The model under review builds one solid part; all positions refer to its coordinate system, in mm. Face numbers are marked on the shaded views. Coordinates: 2 decimals unless noted, no trailing zeros. Write each loop counter-clockwise with the first axis right and the second up, starting at its lowest first coordinate (ties: lowest second). Pieces come first, ordered by that corner, then holes. Notation, with made-up numbers: (28.25, 24.25) - (73.25, 24.25) arc R20 ccw to (73.25, 57.25) - close; hole circle Ø9 at (-4.75, -16.5). An arc over 180 degrees is marked (long way). Put each result on its own line as item: value. Start each with the question number.
Item 1: Consider section D-D on y = 3.5. Give the boundary of the cut face in (x, z).
Item 2: Consider section A-A on y = 1.75. Give the boundary of the cut face in (x, z).
Item 3: To check wall thickness, follow L1, parallel to Y at x = 0, z = 0.5; L2, parallel to X at y = -1, z = 2; L3, parallel to X at y = -0.5, z = 1.5. State the ranges of each line that lie inside material, in increasing order. Write a range as [from, to].
Item 4: For pin 1 (1 mm diameter, centred on y = -2, z = 1, fed in from +X), flat-tipped, find the tip position at first contact; note if it passes through.
Item 5: Consider section B-B on y = 0. Give the boundary of the cut face in (x, z).
Item 6: Mouldability with a two-part tool opening along X and no side actions: class the marked faces 1, 2 and 3 as pulls with the +X half, pulls with the -X half, needs draft (parallel to the pull), parting line crosses it, or undercut.
Item 7: Consider section C-C on x = 17.5. Give the boundary of the cut face in (y, z), then the cut area to 3 significant figures.
```python
from build123d import *

# Parameters (mm, degrees)
BOSS_EXTRUDE1_DEPTH     = 3.556
CUT_EXTRUDE1_DEPTH      = 23.127926609
CUT_EXTRUDE1_DEPTH_BACK = 23.127926609
SKETCH6_R               = 3


with BuildPart() as part:
    # Sketch1 → Boss-Extrude1 (new, symmetric)
    with BuildSketch(Plane.XY):
        with BuildLine():
            Line((-15, 6), (15, 6))
            ThreePointArc((15, 6), (21, 0), (15, -6))
            Line((15, -6), (-15, -6))
            ThreePointArc((-15, -6), (-21, 0), (-15, 6))
        make_face()
    extrude(amount=BOSS_EXTRUDE1_DEPTH, both=True)

    # Sketch6 → Cut-Extrude1 (cut, two sides: drawn at the far end of the back side and taken through both)
    with BuildSketch(Plane(origin=(0, 0, 0), x_dir=(0, 1, 0), z_dir=(-0.500000000000001, 0, 0.866025403784438)).offset(-CUT_EXTRUDE1_DEPTH_BACK)):
        with Locations(Location((0, 0, 0), (0, 0, 90))):
            Circle(SKETCH6_R)
    extrude(amount=CUT_EXTRUDE1_DEPTH + CUT_EXTRUDE1_DEPTH_BACK, mode=Mode.SUBTRACT)


solid = part.part
```
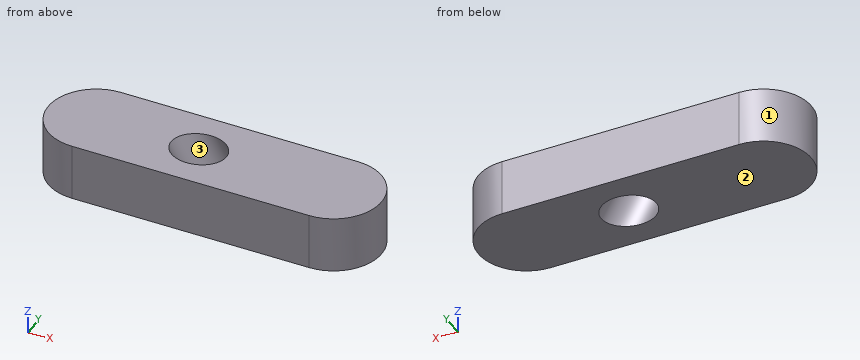
Report:
1. outline: (-19.87, -3.56) - (19.87, -3.56) - (19.87, 3.56) - (-19.87, 3.56) - close
2. outline: (-20.74, -3.56) - (-0.76, -3.56) - (-4.87, 3.56) - (-20.74, 3.56) - close; (0.76, 3.56) - (4.87, -3.56) - (20.74, -3.56) - (20.74, 3.56) - close
3. L1: [-6, -2.99], [2.99, 6]
3. L2: [-20.92, -4.42], [2.11, 20.92]
3. L3: [-20.98, -4.28], [2.55, 20.98]
4. pin 1: x = 20.81
5. outline: (-21, -3.56) - (-1.41, -3.56) - (-5.52, 3.56) - (-21, 3.56) - close; (1.41, 3.56) - (5.52, -3.56) - (21, -3.56) - (21, 3.56) - close
6. face 1: pulls with the -X half
6. face 2: needs draft
6. face 3: undercut
7. outline: (-5.45, -3.56) - (5.45, -3.56) - (5.45, 3.56) - (-5.45, 3.56) - close
7. area: 77.6 mm²
